Check sheet for the modelled part. Datum: model origin and axes. Units: mm. A direction names the side the tool comes from. Coordinates: 2 decimals unless noted, no trailing zeros. Write each loop counter-clockwise with the first axis right and the second up, starting at its lowest first coordinate (ties: lowest second). Pieces come first, ordered by that corner, then holes. Notation, with made-up numbers: (33.5, 84.5) -> (37.5, 84.5) arc R16 ccw to (37.5, 112.5) -> close; hole circle Ø11 at (-1.5, -32.75). An arc over 180 degrees is marked (long way). One line per item, written item: value. Start each with the question number.
1) Sectioned sample at C-C on z = 3.7. Enter the section's corners in (x, y).
2) Sectioned sample at A-A on y = 0.05. Enter the section's corners in (x, z).
3) Scan lines: line 1 along Y through (x, z) = (1.25, 0.45); line 2 along X through (y, z) = (0, 1.75). Record each from-to range of solid material in increasing order. Write a range as [from, to].
4) Draft check along X on faces 1 (the flat face through (6, 0, 2)), 2 (the flat face through (0, 3, 2)), 3 (the flat face through (0, -0.7, 2)). Enter one of: +X half, -X half, draft (parallel to the pull), parting line (faces both ways), or undercut.
5) Set-up check for faces 4 (the flat face through (1.7, 0, 2)), 5 (the flat face through (0, -1, 5)): record each of +Z, -Z, +X, -X, +Y, -Y from which the full face is reachable in a straight line by a thin tool's end or side.
6) Sectioned sample at B-B on x = -1.5. Enter the section's corners in (y, z), plus the area to 3 significant figures.
```python
from build123d import *

# Parameters (mm, degrees)
PAD002_DEPTH               = 5
PAD002_MIRRORED002_2_DEPTH = 5


with BuildPart() as part:
    # Sketch004 → Pad002 (new body)
    with BuildSketch(Plane.XY):
        Polygon((6, 0), (6, 3), (0, 3), (0, 0.7), (1.7, 0.7), (1.7, 0), align=None)
    pad002 = extrude(amount=PAD002_DEPTH)

    # Sketch004 Mirrored002 2 → Pad002 Mirrored002 2 (add)
    with BuildSketch(Plane(origin=(0, 0, 0), x_dir=(-1, 0, 0), z_dir=(0, 0, -1))):
        Polygon((6, 0), (6, 3), (0, 3), (0, 0.7), (1.7, 0.7), (1.7, 0), align=None)
    pad002_mirrored002_2 = extrude(amount=-PAD002_MIRRORED002_2_DEPTH)

    # Mirrored003: Pad002, Pad002 Mirrored002 2 across Sketch004 H_Axis
    add(pad002.mirror(Plane.ZX))
    add(pad002_mirrored002_2.mirror(Plane.ZX))


solid = part.part
```
Answers:
1. outline: (-6, -3) -> (6, -3) -> (6, 3) -> (-6, 3) -> close; hole (-1.7, -0.7) -> (1.7, -0.7) -> (1.7, 0.7) -> (-1.7, 0.7) -> close
2. outline: (-6, 0) -> (-1.7, 0) -> (-1.7, 5) -> (-6, 5) -> close; (1.7, 0) -> (6, 0) -> (6, 5) -> (1.7, 5) -> close
3. line 1: y = [-3, -0.7], [0.7, 3]
3. line 2: x = [-6, -1.7], [1.7, 6]
4. face 1: +X half
4. face 2: draft
4. face 3: undercut
5. face 4: +Z, -Z
5. face 5: +Z, +X, -X, +Y, -Y
6. outline: (-3, 0) -> (-0.7, 0) -> (-0.7, 5) -> (-3, 5) -> close; (0.7, 0) -> (3, 0) -> (3, 5) -> (0.7, 5) -> close
6. area: 23.0 mm2
